Job drawing, mm, ordinate dimensions from the low corner. One solid piece. Give positions to 0.01 mm unless a question says otherwise; leave off trailing zeros. Order: outer loops, then holes, each group sorted by start corner. A loop starts at its lowest first (then second) coordinate and runs counter-clockwise, first axis right, second up.
1. Probe line 1 (X direction, y = 0.25, z = 15.25); line 2 (Z direction, x = 26.75, y = 1.4); line 3 (Z direction, x = 28.5, y = 0.7). List the from-to ranges inside material, lowest first.
2. Slice it at A-A on y = 0.8. List the corners of the cut face in (x, z).
3. Slice it at B-B on z = 6.75. List the corners of the cut face in (x, y), and give its area (3 significant figures).
4. Drop a flat-ended pin along its axis: pin 1 Ø0.8 at (y, z) = (1, 11) entering from -X. Give the stop position or say it passes through.
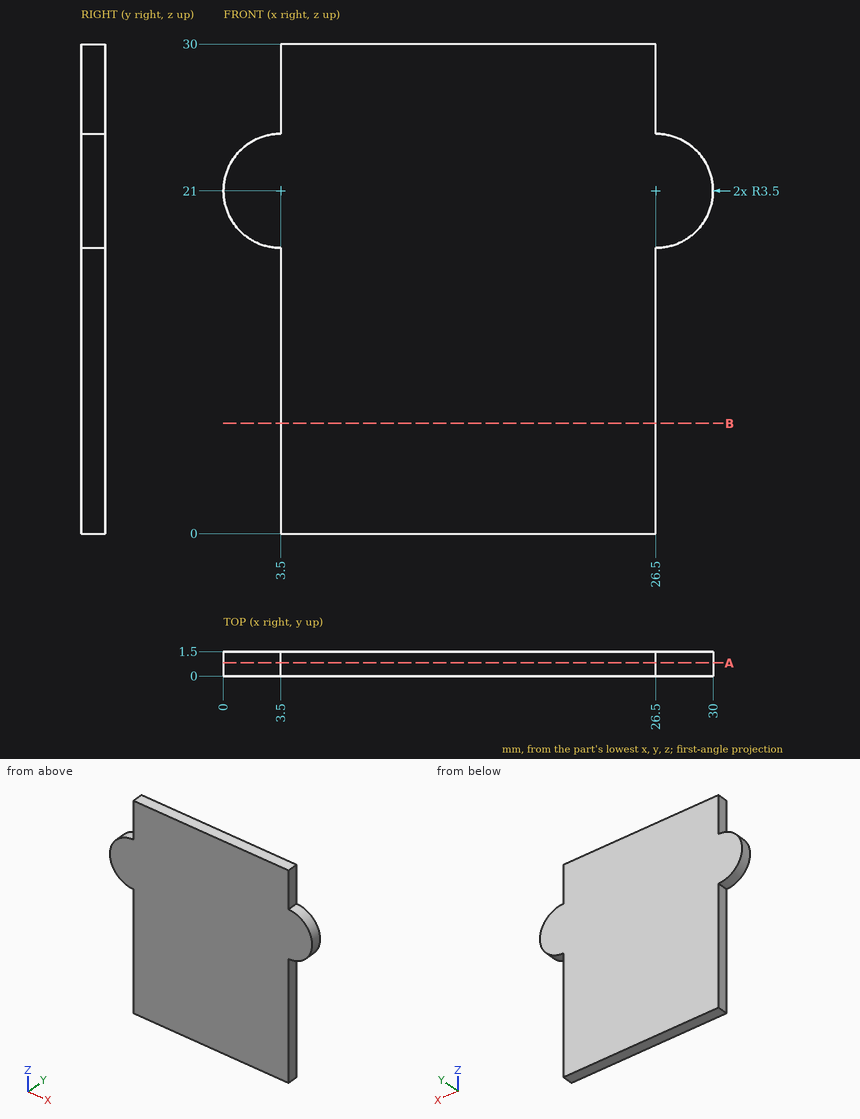
Data:
1. line 1: x = 3.5 to 26.5
1. line 2: z = 17.51 to 24.49
1. line 3: z = 18.13 to 23.87
2. outline: (3.5, 0) - (26.5, 0) - (26.5, 17.5) arc R3.5 ccw to (26.5, 24.5) - (26.5, 30) - (3.5, 30) - (3.5, 24.5) arc R3.5 ccw to (3.5, 17.5) - close
3. outline: (3.5, 0) - (26.5, 0) - (26.5, 1.5) - (3.5, 1.5) - close
3. area: 34.5 mm2
4. pin 1: stops at x = 3.5
